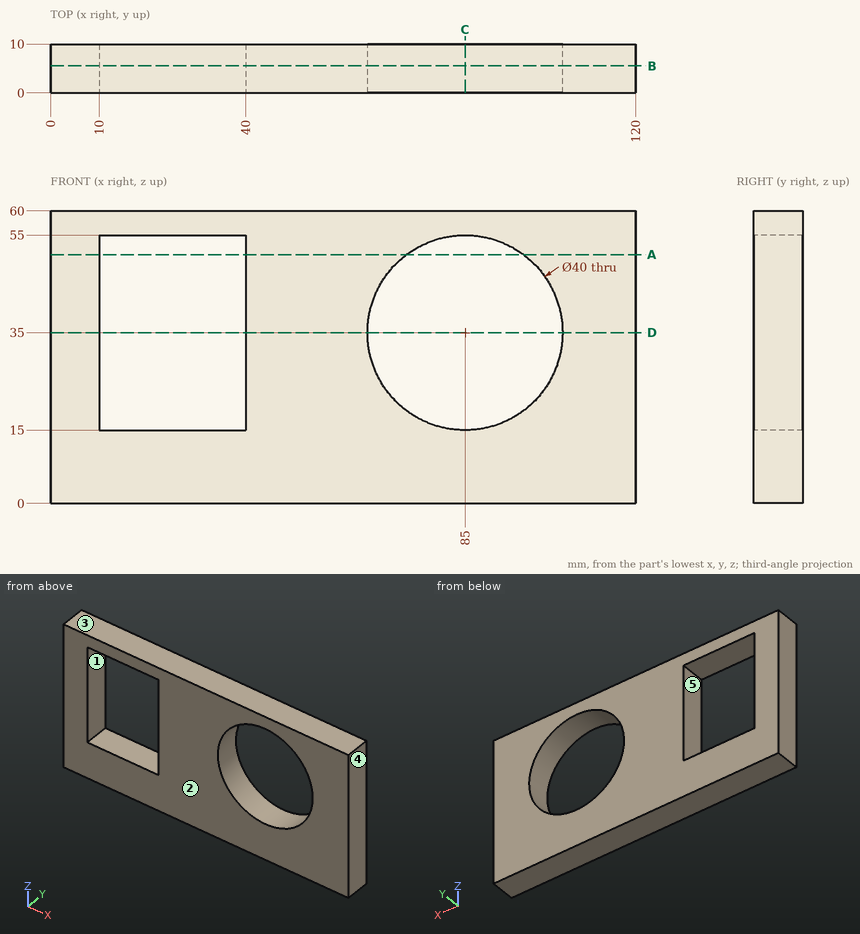
Geometry: see drawing. Coordinates: mm, zero at the bounding-box minimum. A direction names the side the tool comes from. Coordinates: 2 decimals unless noted, no trailing zeros. Loops run counter-clockwise (first coordinate to the right, second up) from the corner with the lowest first, then second, coordinate; pieces in that order, holes last. Notation, with made-up numbers: (67, 5) -> (109, 5) arc R14 cw to (109, 25) -> close; hole circle Ø7 at (59, -16). An arc over 180 degrees is marked (long way). Write item = value, one per line. Start each with the question number.
Item 1: Material intervals for line 1 (X direction, y = 5.5, z = 35); line 2 (X direction, y = 5.75, z = 53); line 3 (Z direction, x = 78, y = 8) (3 decimals), sorted ascending.
Item 2: Cut plane D-D, the plane z = 35. Return loops of the section in (x, y).
Item 3: Reachability of the marked faces 4 and 5 from +Z, -Z, +X, -X, +Y, -Y: full face, straight path, thin tool, end or side. Return the list, or none.
Item 4: First-contact query: P1, Ø10, axis at x = 44, z = 43.5, coming from the -Y side. Flat tip, straight axial feed; report the tip coordinate or a pass-through.
Item 5: Mould query, pull axis Z, two halves, no side actions, for the marked faces 1, 2 and 3. Classes: pulls with the +Z half, pulls with the -Z half, needs draft (parallel to the pull), parting line crosses it, or undercut.
Item 6: Cut plane B-B, the plane y = 5.5. Return loops of the section in (x, z).
Item 7: Cut plane A-A, the plane z = 51. Return loops of the section in (x, y), plus the area to 3 significant figures.
Item 8: Cut plane C-C, the plane x = 85. Return loops of the section in (y, z), plus the area to 3 significant figures.
Ans:
q1.line_1 = 0 to 10, 40 to 65, 105 to 120
q1.line_2 = 0 to 10, 40 to 76.28, 93.72 to 120
q1.line_3 = 0 to 16.265, 53.735 to 60
q2.outline = (0, 0) -> (10, 0) -> (10, 10) -> (0, 10) -> close; (40, 0) -> (65, 0) -> (65, 10) -> (40, 10) -> close; (105, 0) -> (120, 0) -> (120, 10) -> (105, 10) -> close
q3.face_4 = +Z, -Z, +X, +Y, -Y
q3.face_5 = +Y, -Y
q4.P1 = 0
q5.face_1 = undercut
q5.face_2 = needs draft
q5.face_3 = pulls with the +Z half
q6.outline = (0, 0) -> (120, 0) -> (120, 60) -> (0, 60) -> close; hole (10, 15) -> (40, 15) -> (40, 55) -> (10, 55) -> close; hole circle Ø40 at (85, 35)
q7.outline = (0, 0) -> (10, 0) -> (10, 10) -> (0, 10) -> close; (40, 0) -> (73, 0) -> (73, 10) -> (40, 10) -> close; (97, 0) -> (120, 0) -> (120, 10) -> (97, 10) -> close
q7.area = 660 mm²
q8.outline = (0, 0) -> (10, 0) -> (10, 15) -> (0, 15) -> close; (0, 55) -> (10, 55) -> (10, 60) -> (0, 60) -> close
q8.area = 200 mm²
